```python
from build123d import *

# Parameters (mm, degrees)
PANEL_W                      = 1000
PANEL_H                      = 284
PANEL_PLY_DEPTH              = 12
SKETCH2_W                    = 12
SKETCH2_H                    = 284
VERTICAL_HOUSING_CUT_DEPTH   = 4
SKETCH3_W                    = 393
SKETCH3_H                    = 12
HORIZONTAL_HOUSING_CUT_DEPTH = 4


with BuildPart() as part:
    # Panel → Panel Ply (new body)
    with BuildSketch(Plane.XY):
        with Locations((500, 142)):
            Rectangle(PANEL_W, PANEL_H)
    extrude(amount=PANEL_PLY_DEPTH)

    # Sketch2 → Vertical Housing Cut (cut)
    with BuildSketch(Plane.XY.offset(12)):
        with Locations((6, 142)):
            Rectangle(SKETCH2_W, SKETCH2_H)
        with Locations((994, 142)):
            Rectangle(SKETCH2_W, SKETCH2_H)
        with Locations((411, 142)):
            Rectangle(SKETCH2_W, SKETCH2_H)
        with Locations((589, 142)):
            Rectangle(SKETCH2_W, SKETCH2_H)
    extrude(amount=-VERTICAL_HOUSING_CUT_DEPTH, mode=Mode.SUBTRACT)

    # Sketch3 → Horizontal Housing Cut (cut)
    with BuildSketch(Plane.XY.offset(12)):
        with Locations((208.5, 142)):
            Rectangle(SKETCH3_W, SKETCH3_H)
        with Locations((791.5, 142)):
            Rectangle(SKETCH3_W, SKETCH3_H)
    extrude(amount=-HORIZONTAL_HOUSING_CUT_DEPTH, mode=Mode.SUBTRACT)


solid = part.part
```
Model file for the job. Use its own axes, mm. Coordinates: 2 decimals unless noted, no trailing zeros. Order: outer loops, then holes, each group sorted by start corner. A loop starts at its lowest first (then second) coordinate and runs counter-clockwise, first axis right, second up. Notation, with made-up numbers: (-31.5, 54) -> (18.5, 54) arc R17 cw to (18.5, 80) -> close; hole circle Ø11 at (88.25, 29.5). An arc over 180 degrees is marked (long way). Answer as a JSON object with one key per item and string values. Group by question number.
1) Flat gauge pins, fed straight in: pin 1 (3 mm diameter, centred on y = 66, z = 10, fed in from -X); pin 2 (2 mm diameter, centred on y = 93.5, z = 9.5, fed in from +X). Where does each tip first touch, or does it go through?
2) Drill centre lines: L1, parallel to X at y = 48.5, z = 9.25; L2, parallel to Y at x = 144, z = 9. Where is each one in solid material? Low to high.
3) Pull direction Y, two halves, no side cores. Call faces 1 (the face through (208, 143, 8)), 2 (the face through (493, 144, 0)): +Y half, -Y half, draft (parallel to the pull), parting line (faces both ways), or undercut.
4) Cut at A-A, the plane y = 220.5. Write the cut outline in (x, z).
Check values:
{
 "1": {"pin 1": "stops at x = 12", "pin 2": "stops at x = 988"},
 "2": {"L1": "x = 12 to 405, 417 to 583, 595 to 988", "L2": "y = 0 to 136, 148 to 284"},
 "3": {"face 1": "undercut", "face 2": "draft"},
 "4": {"outline": "(0, 0) -> (1000, 0) -> (1000, 8) -> (988, 8) -> (988, 12) -> (595, 12) -> (595, 8) -> (583, 8) -> (583, 12) -> (417, 12) -> (417, 8) -> (405, 8) -> (405, 12) -> (12, 12) -> (12, 8) -> (0, 8) -> close"}
}
